```python
from build123d import *

# Parameters (mm, degrees)
SKETCH1_R                    = 14
BOSS_EXTRUDE1_DEPTH          = 36.4
SKETCH2_R                    = 5
BOSS_EXTRUDE2_DEPTH          = 0.5
SKETCH3_R                    = 1.5875
BOSS_EXTRUDE3_DEPTH          = 10.5
F_3_0_3_DIAMETER_HOLE1_D     = 3
F_3_0_3_DIAMETER_HOLE1_DEPTH = 4
F_3_0_3_DIAMETER_HOLE1_TIP   = 0.901290929


with BuildPart() as part:
    # Sketch1 → Boss-Extrude1 (new body)
    with BuildSketch(Plane.XY):
        Circle(SKETCH1_R)
    extrude(amount=BOSS_EXTRUDE1_DEPTH)

    # Sketch2 → Boss-Extrude2 (add)
    with BuildSketch(Plane.XY.offset(36.4)):
        Circle(SKETCH2_R)
    extrude(amount=BOSS_EXTRUDE2_DEPTH)

    # Sketch3 → Boss-Extrude3 (add)
    with BuildSketch(Plane.XY.offset(36.9)):
        with Locations(Location((0, 0, 0), (0, 0, 180))):
            Circle(SKETCH3_R)
    extrude(amount=BOSS_EXTRUDE3_DEPTH)

    # Ø3.0 (3) Diameter Hole1
    with Locations(Plane.XY.offset(36.4)):
        with Locations((0, 9.5), (0, -9.5), (8, 0), (-8, 0)):
            Hole(F_3_0_3_DIAMETER_HOLE1_D / 2, depth=F_3_0_3_DIAMETER_HOLE1_DEPTH)
            with Locations((0, 0, -(F_3_0_3_DIAMETER_HOLE1_DEPTH + F_3_0_3_DIAMETER_HOLE1_TIP / 2))):  # 118° drill point
                Cone(0, F_3_0_3_DIAMETER_HOLE1_D / 2, F_3_0_3_DIAMETER_HOLE1_TIP, mode=Mode.SUBTRACT)


solid = part.part
```
For this review, take the finished solid that the model builds, in its own axes (mm). A direction names the side the tool comes from. Give positions to 0.01 mm unless a question says otherwise; leave off trailing zeros. Write each loop counter-clockwise with the first axis right and the second up, starting at its lowest first coordinate (ties: lowest second). Pieces come first, ordered by that corner, then holes. Notation, with made-up numbers: M -24,8 L 35,8 A28 ccw 35,41 Z; hole C 56.25,9 d5. An arc over 180 degrees is marked long. Answer as a JSON object with one key per item and string values. Group by question number.
Item 1: Consider section A-A on z = 33.5. Write out the cut boundary in (x, y).
Item 2: For pin 1 Ø1 at (y, z) = (3, 38.5) entering from +X; pin 2 Ø6 at (y, z) = (5, 28.5) entering from -X; pin 3 Ø2.5 at (x, y) = (0, 9.5) entering from +Z; pin 4 Ø2 at (y, z) = (9, 24.5) entering from +X, all flat-tipped, find the tip position at first contact; note any pin that passes through.
Item 3: Draft analysis for pull direction Y (two halves, no side actions). For faces 3 (the flat face through (0, -6, 36.4)), 4 (the conical face through (7.74, 0.011, 31.655)), 5 (the cylindrical face through (-0.73, 1.41, 42.08)), state which applies: +Y half, -Y half, draft (parallel to the pull), parting line (faces both ways), or undercut.
Item 4: Consider section B-B on x = 3.75. Write out the cut boundary in (y, z), plus the area to 3 significant figures.
Item 5: For probe 1 along Y at (x, z) = (0, 35.4); probe 2 along Z at (x, y) = (4.25, 2); probe 3 along Z at (x, y) = (10, 5.5), list the stretches that pass through material, from the lowest coordinate up. Write a range as [from, to].
Item 6: Consider section D-D on z = 10.5. Write out the cut boundary in (x, y), plus the area to 3 significant figures.
Item 7: Tool access review of faces 1 (the cylindrical face through (9.5, 0.07, 34.37)), 2 (the flat face through (0, 0, 0)): name each direction out of +Z, -Z, +X, -X, +Y, -Y from which nothing blocks a thin tool from reaching the whole face with its end or side.
Item 8: Consider section C-C on y = 12. Write out the cut boundary in (x, z), plus the area to 3 significant figures.
Check result:
{
 "1": {"outline": "C 0,0 d28; hole C -8,0 d3; hole C 0,-9.5 d3; hole C 0,9.5 d3; hole C 8,0 d3"},
 "2": {"pin 1": "passes through", "pin 2": "stops at x = -13.86", "pin 3": "stops at z = 32.25", "pin 4": "stops at x = 11.49"},
 "3": {"face 3": "draft", "face 4": "undercut", "face 5": "parting line"},
 "4": {"outline": "M -13.49,0 L 13.49,0 L 13.49,36.4 L 3.31,36.4 L 3.31,36.9 L -3.31,36.9 L -3.31,36.4 L -13.49,36.4 Z", "area": "985 mm^2"},
 "5": {"probe 1": "y = [-14, -11], [-8, 8], [11, 14]", "probe 2": "z = [0, 36.9]", "probe 3": "z = [0, 36.4]"},
 "6": {"outline": "C 0,0 d28", "area": "616 mm^2"},
 "7": {"face 1": "+Z", "face 2": "-Z, +X, -X, +Y, -Y"},
 "8": {"outline": "M -7.21,0 L 7.21,0 L 7.21,36.4 L -7.21,36.4 Z", "area": "525 mm^2"}
}
